from build123d import *

# Parameters (mm, degrees)
BOSS_EXTRUDE1_DEPTH = 98.705
BOSS_EXTRUDE2_START = 7
SKETCH5_W           = 150
SKETCH5_H           = 132.5
BOSS_EXTRUDE2_DEPTH = 7
FILLET1_R           = 10
CUT_EXTRUDE1_DEPTH  = 5.099


with BuildPart() as part:
    # Sketch1 → Boss-Extrude1 (new body)
    with BuildSketch(Plane.XY):
        with BuildLine():
            Line((-54.25, 62.25), (54.25, 62.25))
            ThreePointArc((54.25, 62.25), (56.371320344, 61.371320344), (57.25, 59.25))
            Line((57.25, 59.25), (57.25, -59.25))
            ThreePointArc((57.25, -59.25), (56.371320344, -61.371320344), (54.25, -62.25))
            Line((54.25, -62.25), (-54.25, -62.25))
            ThreePointArc((-54.25, -62.25), (-56.371320344, -61.371320344), (-57.25, -59.25))
            Line((-57.25, -59.25), (-57.25, 59.25))
            ThreePointArc((-57.25, 59.25), (-56.371320344, 61.371320344), (-54.25, 62.25))
        make_face()
        with BuildLine():
            Line((-55.25, 59.25), (-55.25, -59.25))
            ThreePointArc((-55.25, -59.25), (-54.957106781, -59.957106781), (-54.25, -60.25))
            Line((-54.25, -60.25), (54.25, -60.25))
            ThreePointArc((54.25, -60.25), (54.957106781, -59.957106781), (55.25, -59.25))
            Line((55.25, -59.25), (55.25, 59.25))
            ThreePointArc((55.25, 59.25), (54.957106781, 59.957106781), (54.25, 60.25))
            Line((54.25, 60.25), (-54.25, 60.25))
            ThreePointArc((-54.25, 60.25), (-54.957106781, 59.957106781), (-55.25, 59.25))
        make_face(mode=Mode.SUBTRACT)
    extrude(amount=-BOSS_EXTRUDE1_DEPTH)

    # Sketch5 → Boss-Extrude2 (add)
    with BuildSketch(Plane.XY.offset(BOSS_EXTRUDE2_START)):
        Rectangle(SKETCH5_W, SKETCH5_H)
        with BuildLine():
            Line((-54.25, -60.25), (54.25, -60.25))
            ThreePointArc((54.25, -60.25), (54.957106781, -59.957106781), (55.25, -59.25))
            Line((55.25, -59.25), (55.25, 59.25))
            ThreePointArc((55.25, 59.25), (54.957106781, 59.957106781), (54.25, 60.25))
            Line((54.25, 60.25), (-54.25, 60.25))
            ThreePointArc((-54.25, 60.25), (-54.957106781, 59.957106781), (-55.25, 59.25))
            Line((-55.25, 59.25), (-55.25, -59.25))
            ThreePointArc((-55.25, -59.25), (-54.957106781, -59.957106781), (-54.25, -60.25))
        make_face(mode=Mode.SUBTRACT)
    extrude(amount=-BOSS_EXTRUDE2_DEPTH)

    # Fillet1
    fillet1_edges = [part.edges().sort_by_distance(p)[0] for p in [
        (-75, 66.25, 3.5),
        (-75, -66.25, 3.5),
        (75, -66.25, 3.5),
        (75, 66.25, 3.5),
    ]]
    fillet(fillet1_edges, radius=FILLET1_R)

    # Sketch6 → Cut-Extrude1 (cut)
    with BuildSketch(Plane.XY.offset(7)):
        with BuildLine():
            Line((73, -56.25), (73, 56.25))
            ThreePointArc((73, 56.25), (70.656854249, 61.906854249), (65, 64.25))
            Line((65, 64.25), (-65, 64.25))
            ThreePointArc((-65, 64.25), (-70.656854249, 61.906854249), (-73, 56.25))
            Line((-73, 56.25), (-73, -56.25))
            ThreePointArc((-73, -56.25), (-70.656854249, -61.906854249), (-65, -64.25))
            Line((-65, -64.25), (65, -64.25))
            ThreePointArc((65, -64.25), (70.656854249, -61.906854249), (73, -56.25))
        make_face()
    extrude(amount=-CUT_EXTRUDE1_DEPTH, mode=Mode.SUBTRACT)


solid = part.part
Input: part model. Units: mm. Frame: model coordinates. A direction names the side the tool comes from. Coordinates: 2 decimals unless noted, no trailing zeros. Loops run counter-clockwise (first coordinate to the right, second up) from the corner with the lowest first, then second, coordinate; pieces in that order, holes last. Notation, with made-up numbers: (86.25, 25) - (117.25, 25) arc R16 ccw to (117.25, 43) - close; hole circle Ø11 at (20, -14.5). An arc over 180 degrees is marked (long way). Answer in a Markdown table with one row per item. Add a question column.
Item 1: Mould query, pull axis Y, two halves, no side actions, for faces 6 (the flat face through (-1, 66.25, 4)), 7 (the flat face through (73, -1, 4)), 8 (the flat face through (-75, -1, 4)). Classes: released by +Y, released by -Y, zero draft, split by the parting line, or undercut.
Item 2: Access query for faces 1 (the flat face through (1, -62.25, -49)), 2 (the flat face through (57.25, 1, -49)), 3 (the flat face through (-60, -4, 1.901)), 4 (the cylindrical face through (-72.15, 63.24, 3.45)), 5 (the flat face through (-55.25, 1, -48)). Directions: +Z, -Z, +X, -X, +Y, -Y. A direction counts if a zero-diameter tool reaches every point of the face in a straight line with its end or side. Return the directions, or none.
Item 3: Section query D-D on x = -60. Return the cut outline in (y, z), then the cut area to 3 significant figures.
Item 4: Section query C-C on y = -41.5. Return the cut outline in (x, z) (3 decimals), then the cut area to 3 significant figures.
Item 5: Section query A-A on x = 33.5. Return the cut outline in (y, z) (3 decimals), then the cut area to 3 significant figures.
Item 6: Line query: line 1 along X through (y, z) = (6, -41); line 2 along Y through (x, z) = (22, -89); line 3 along X through (y, z) = (25, 0.5). Output: solid intervals per line, ascending. Write a range as [from, to].
Item 7: Section query B-B on z = -38. Return the cut outline in (x, y).
Item 8: Contact query for flat-ended pins moving along their axis: P1, Ø5, axis at x = -22.5, z = -70.5, coming from the -Y side; P2, Ø5, axis at y = 12, z = -66, coming from the -X side; P3, Ø3, axis at y = 13, z = -7.5, coming from the +X side; P4, Ø2, axis at x = 53, y = 2.5, coming from the -Z side. Output: stop coordinate, or through.
Recorded:
| question | item | result |
|---|---|---|
| 1 | face 6 | released by +Y |
| 1 | face 7 | undercut |
| 1 | face 8 | zero draft |
| 2 | face 1 | -Z, +X, -X, -Y |
| 2 | face 2 | -Z, +X, +Y, -Y |
| 2 | face 3 | +Z |
| 2 | face 4 | +Z, -Z, -X, +Y |
| 2 | face 5 | +Z, -Z |
| 3 | outline | (-66.25, 0) - (66.25, 0) - (66.25, 7) - (64.25, 7) - (64.25, 1.9) - (-64.25, 1.9) - (-64.25, 7) - (-66.25, 7) - close |
| 3 | area | 272 mm^2 |
| 4 | outline | (-75, 0) - (-57.25, 0) - (-57.25, -98.705) - (-55.25, -98.705) - (-55.25, 1.901) - (-73, 1.901) - (-73, 7) - (-75, 7) - close; (55.25, -98.705) - (57.25, -98.705) - (57.25, 0) - (75, 0) - (75, 7) - (73, 7) - (73, 1.901) - (55.25, 1.901) - close |
| 4 | area | 490 mm^2 |
| 5 | outline | (-66.25, 0) - (-62.25, 0) - (-62.25, -98.705) - (-60.25, -98.705) - (-60.25, 1.901) - (-64.25, 1.901) - (-64.25, 7) - (-66.25, 7) - close; (60.25, -98.705) - (62.25, -98.705) - (62.25, 0) - (66.25, 0) - (66.25, 7) - (64.25, 7) - (64.25, 1.901) - (60.25, 1.901) - close |
| 5 | area | 438 mm^2 |
| 6 | line 1 | [-57.25, -55.25], [55.25, 57.25] |
| 6 | line 2 | [-62.25, -60.25], [60.25, 62.25] |
| 6 | line 3 | [-75, -55.25], [55.25, 75] |
| 7 | outline | (-57.25, -59.25) arc R3 ccw to (-54.25, -62.25) - (54.25, -62.25) arc R3 ccw to (57.25, -59.25) - (57.25, 59.25) arc R3 ccw to (54.25, 62.25) - (-54.25, 62.25) arc R3 ccw to (-57.25, 59.25) - close; hole (-55.25, -59.25) arc R1 ccw to (-54.25, -60.25) - (54.25, -60.25) arc R1 ccw to (55.25, -59.25) - (55.25, 59.25) arc R1 ccw to (54.25, 60.25) - (-54.25, 60.25) arc R1 ccw to (-55.25, 59.25) - close |
| 8 | P1 | y = -62.25 |
| 8 | P2 | x = -57.25 |
| 8 | P3 | x = 57.25 |
| 8 | P4 | through |
